Source: CAD feature listing. Evaluate the final solid. Frame: model axes, mm. A direction names the side the tool comes from. Give positions to 0.01 mm unless a question says otherwise; leave off trailing zeros. Loops run counter-clockwise (first coordinate to the right, second up) from the corner with the lowest first, then second, coordinate; pieces in that order, holes last. Notation, with made-up numbers: M 71.25,16 L 76.25,16 A24 cw 76.25,35 Z; hole C 12.25,59 d7. An arc over 180 degrees is marked long. Answer in a Markdown table with one row per item.
```python
from build123d import *

# Parameters (mm, degrees)
PAD011_DEPTH       = 0.5
SKETCH009_R        = 1.6
SKETCH009_R_2      = 1.2
POCKET012014_DEPTH = 0.501
SKETCH010_R        = 2.8
SKETCH010_R_2      = 1.6
PAD012_DEPTH       = 2.5
SKETCH011_R        = 1.1
PAD013_DEPTH       = 1.5


with BuildPart() as part:
    # Sketch008 → Pad011 (new body)
    with BuildSketch(Plane.XY.offset(9)):
        Polygon((18.25, -36.75), (18.25, 36.75), (6.75, 36.75), (6.75, 23.75), (-6.25, 23.75), (-6.25, 36.75), (-18.25, 36.75), (-18.25, -36.75), (-7.25, -36.75), (-7.25, -30.75), (4.75, -30.75), (4.75, -36.75), align=None)
    extrude(amount=PAD011_DEPTH)

    # Sketch009 → Pocket012014 (cut, through all)
    with BuildSketch(Plane.XY.offset(9.5)):
        with Locations((-9.75, 29.25)):
            Circle(SKETCH009_R)
        with Locations((16.75, 29.25)):
            Circle(SKETCH009_R)
        with Locations((9.75, 29.45)):
            Circle(SKETCH009_R_2)
    extrude(amount=-POCKET012014_DEPTH, mode=Mode.SUBTRACT)

    # Sketch010 → Pad012 (new body)
    with BuildSketch(Plane.XY.offset(9.5)):
        with Locations((-9.75, 29.25)):
            Circle(SKETCH010_R)
        with Locations((-9.75, 29.25)):
            Circle(SKETCH010_R_2, mode=Mode.SUBTRACT)
        with Locations((-9.75, -11.75)):
            Circle(SKETCH010_R)
        with BuildLine():
            ThreePointArc((18.25, 29.806776), (15.15, 29.25), (18.25, 28.693224))
            Line((18.25, 28.693224), (18.25, 26.885682))
            ThreePointArc((18.25, 31.614318), (13.95, 29.25), (18.25, 26.885682))
            Line((18.25, 31.614318), (18.25, 29.806776))
        make_face()
        with BuildLine():
            ThreePointArc((18.25, -9.385682), (13.95, -11.75), (18.25, -14.114318))
            Line((18.25, -9.385682), (18.25, -14.114318))
        make_face()
    extrude(amount=PAD012_DEPTH)

    # Sketch011 → Pad013 (new body)
    with BuildSketch(Plane.XY.offset(12)):
        with Locations((-9.75, -11.75)):
            Circle(SKETCH011_R)
        with Locations((16.75, -11.75)):
            Circle(SKETCH011_R)
    extrude(amount=PAD013_DEPTH)


solid = part.part
```
1) Section D-D, the plane y = 6. Return loops of the section in (x, z).
Reply:
| item | result |
|---|---|
| outline | M -18.25,9 L 18.25,9 L 18.25,9.5 L -18.25,9.5 Z |
2) Material intervals for L1, parallel to Y at x = 16, z = 11.3; L2, parallel to Y at x = -9.75, z = 9.25; L3, parallel to Z at x = -13, y = 10.5, sorted ascending.
Reply:
| item | result |
|---|---|
| L1 | y = -14.45 to -9.05, 26.55 to 27.84, 30.66 to 31.95 |
| L2 | y = -36.75 to 27.65, 30.85 to 36.75 |
| L3 | z = 9 to 9.5 |
3) Section A-A, the plane x = 16.75. Return loops of the section in (y, z), then the cut area to 4 significant figures.
Reply:
| item | result |
|---|---|
| outline | M -36.75,9 L 27.65,9 L 27.65,12 L 26.45,12 L 26.45,9.5 L -8.95,9.5 L -8.95,12 L -10.65,12 L -10.65,13.5 L -12.85,13.5 L -12.85,12 L -14.55,12 L -14.55,9.5 L -36.75,9.5 Z; M 30.85,9 L 36.75,9 L 36.75,9.5 L 32.05,9.5 L 32.05,12 L 30.85,12 Z |
| area | 58.45 mm² |
4) Section C-C, the plane y = -11.75. Return loops of the section in (x, z), then the cut area to 3 significant figures.
Reply:
| item | result |
|---|---|
| outline | M -18.25,9 L 18.25,9 L 18.25,12 L 17.85,12 L 17.85,13.5 L 15.65,13.5 L 15.65,12 L 13.95,12 L 13.95,9.5 L -6.95,9.5 L -6.95,12 L -8.65,12 L -8.65,13.5 L -10.85,13.5 L -10.85,12 L -12.55,12 L -12.55,9.5 L -18.25,9.5 Z |
| area | 49.6 mm² |
5) Pin query (flat end, axial travel): pin 1 Ø4 at (x, y) = (-9.75, 29.25) entering from +Z; pin 2 Ø4.5 at (x, y) = (-9, -10.5) entering from +Z; pin 3 Ø0.6 at (x, z) = (-3.5, 9) entering from -Y; pin 4 Ø1.4 at (x, y) = (9.75, 29.45) entering from -Z. Return the tip coordinate at first contact, or that it passes through.
Reply:
| item | result |
|---|---|
| pin 1 | stops at z = 12 |
| pin 2 | stops at z = 13.5 |
| pin 3 | stops at y = -30.75 |
| pin 4 | passes through |
6) Set-up query: faces 1 (the flat face through (15, 29, 12)), 2 (the cylindrical face through (8.55, 29.5, 9.25)), 3 (the cylindrical face through (13.95, 29.33, 10.73)). Return all of +Z, -Z, +X, -X, +Y, -Y with unobstructed straight access to the full face (end or side cutting, diameter ignored); none if empty.
Reply:
| item | result |
|---|---|
| face 1 | +Z, +X, -X, +Y |
| face 2 | +Z, -Z |
| face 3 | +Z |
7) Pull-direction query (Y, two-part tool) for faces 4 (the cylindrical face through (13.95, -11.67, 10.73)), 5 (the cylindrical face through (15.88, -12.42, 12.74)), 6 (the flat face through (18.25, 31.69, 9.15)); classes: released by +Y, released by -Y, zero draft, split by the parting line, or undercut.
Reply:
| item | result |
|---|---|
| face 4 | undercut |
| face 5 | split by the parting line |
| face 6 | zero draft |
8) Section B-B, the plane x = 9.75. Return loops of the section in (y, z), then the cut area to 4 significant figures.
Reply:
| item | result |
|---|---|
| outline | M -36.75,9 L 28.25,9 L 28.25,9.5 L -36.75,9.5 Z; M 30.65,9 L 36.75,9 L 36.75,9.5 L 30.65,9.5 Z |
| area | 35.55 mm² |
